from build123d import *

# Parameters (mm, degrees)
SKETCH1_R           = 1.524
BOSS_EXTRUDE1_DEPTH = 34.798
SKETCH1_3_R         = 1.524
BOSS_EXTRUDE2_DEPTH = 6.096
CUT_EXTRUDE1_START  = 34.798
SKETCH1_4_R         = 1.524
CUT_EXTRUDE1_DEPTH  = 6.096


with BuildPart() as part:
    # Sketch1 → Boss-Extrude1 (new body)
    with BuildSketch(Plane(origin=(0, 0, 0), x_dir=(1, 0, 0), z_dir=(0, 1, 0))):
        Polygon((-2.794, -1.613116652), (0, -3.226233304), (2.794, -1.613116652), (2.794, 1.613116652), (0, 3.226233304), (-2.794, 1.613116652), align=None)
        Circle(SKETCH1_R, mode=Mode.SUBTRACT)
        Circle(SKETCH1_R)
    extrude(amount=BOSS_EXTRUDE1_DEPTH)

    # Sketch1<3> → Boss-Extrude2 (add)
    with BuildSketch(Plane(origin=(0, 0, 0), x_dir=(1, 0, 0), z_dir=(0, 1, 0))):
        with Locations(Location((0, 0, 0), (0, 0, 270))):
            Circle(SKETCH1_3_R)
    extrude(amount=-BOSS_EXTRUDE2_DEPTH)

    # Sketch1<4> → Cut-Extrude1 (cut)
    with BuildSketch(Plane(origin=(0, 0, 0), x_dir=(1, 0, 0), z_dir=(0, 1, 0)).offset(CUT_EXTRUDE1_START)):
        with Locations(Location((0, 0, 0), (0, 0, 270))):
            Circle(SKETCH1_4_R)
    extrude(amount=-CUT_EXTRUDE1_DEPTH, mode=Mode.SUBTRACT)


solid = part.part
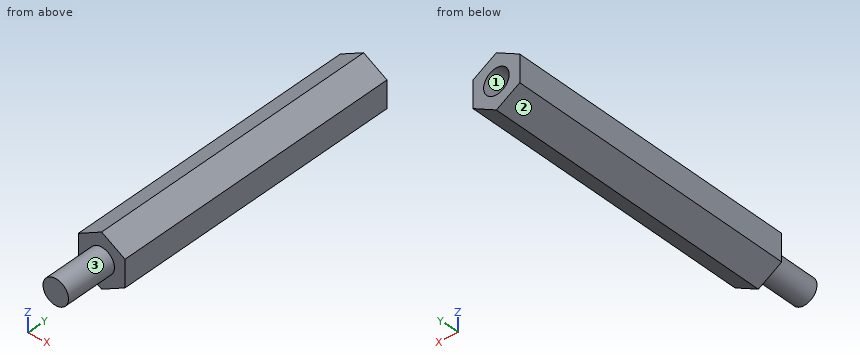
Work out the finished part from the listing and answer in its coordinate system (mm). Face numbers are marked on the shaded views. Give positions to 0.01 mm unless a question says otherwise; leave off trailing zeros. Write each loop counter-clockwise with the first axis right and the second up, starting at its lowest first coordinate (ties: lowest second). Pieces come first, ordered by that corner, then holes. Notation, with made-up numbers: (-10, -4.75) - (47, -4.75) arc R11 ccw to (47, 8.25) - close; hole circle Ø8 at (-37, -3). An arc over 180 degrees is marked (long way). One line per item, written item: value. Start each with the question number.
1. Find section D-D (x = 1.95). Write down the section's boundary in (y, z).
2. For a pull along Z with two mould halves and no side action, classify the marked faces 1, 2 and 3 as +Z half, -Z half, draft (parallel to the pull), parting line (faces both ways), or undercut.
3. Find section C-C (y = 13.5). Write down the section's boundary in (x, z).
4. Find section A-A (z = 0). Write down the section's boundary in (x, y).
5. Consider probe 1 along X at (y, z) = (30.75, 0); probe 2 along Y at (x, z) = (-1.25, -2); probe 3 along Z at (x, y) = (-0.85, 32.5). Determine where each line is inside the solid, lowest interval first.
6. Find section B-B (x = -0.65). Write down the section's boundary in (y, z).
Geometry results:
1. outline: (0, -2.1) - (34.8, -2.1) - (34.8, 2.1) - (0, 2.1) - close
2. face 1: undercut
2. face 2: -Z half
2. face 3: parting line
3. outline: (-2.79, -1.61) - (0, -3.23) - (2.79, -1.61) - (2.79, 1.61) - (0, 3.23) - (-2.79, 1.61) - close
4. outline: (-2.79, 0) - (-1.52, 0) - (-1.52, -6.1) - (1.52, -6.1) - (1.52, 0) - (2.79, 0) - (2.79, 34.8) - (1.52, 34.8) - (1.52, 28.7) - (-1.52, 28.7) - (-1.52, 34.8) - (-2.79, 34.8) - close
5. probe 1: -2.79 to -1.52, 1.52 to 2.79
5. probe 2: 0 to 34.8
5. probe 3: -2.74 to -1.26, 1.26 to 2.74
6. outline: (-6.1, -1.38) - (0, -1.38) - (0, -2.85) - (34.8, -2.85) - (34.8, -1.38) - (28.7, -1.38) - (28.7, 1.38) - (34.8, 1.38) - (34.8, 2.85) - (0, 2.85) - (0, 1.38) - (-6.1, 1.38) - close
